The drawing under review shows one solid part. Ordinate dimensions are in mm from its lowest x, y, z. A direction names the side the tool comes from. Coordinates: 2 decimals unless noted, no trailing zeros. Order: outer loops, then holes, each group sorted by start corner. A loop starts at its lowest first (then second) coordinate and runs counter-clockwise, first axis right, second up. Notation, with made-up numbers: (88, -9.5) -> (101, -9.5) arc R27 ccw to (101, 7.5) -> close; hole circle Ø4 at (50.25, 45). An arc over 180 degrees is marked (long way). Write item = value, one per line.
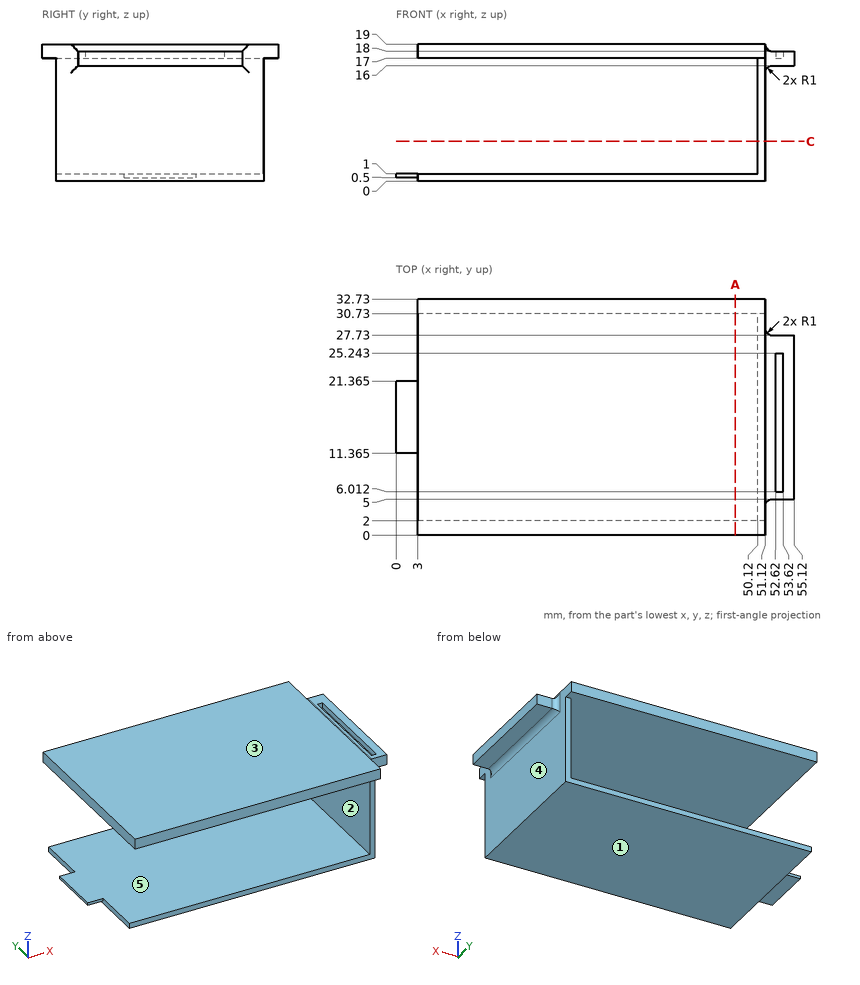
(1) For L1, parallel to Z at x = 11.5, y = 3; L2, parallel to X at y = 23.5, z = 7.75; L3, parallel to Z at x = 52, y = 14, list the stretches that pass through material, from the lowest coordinate up.
Report:
L1 = 0 to 1, 17 to 19
L2 = 50.12 to 51.12
L3 = 15.99 to 18.01
(2) For the marked faces 1 and 2, list the 3-axis set-ups (+Z, -Z, +X, -X, +Y, -Y) from which the entire face can be reached by the end or side of a thin tool; tool diameter is ignored.
Report:
face_1 = -Z, +X, -X, +Y, -Y
face_2 = -X, +Y, -Y
(3) Insertion check: pin 1 (1 mm diameter, centred on y = 21, z = 13.5, fed in from -X); pin 2 (0.5 mm diameter, centred on x = 53, z = 17.5, fed in from +Y); pin 3 (1.1 mm diameter, centred on x = 53, z = 17.5, fed in from -Y); pin 4 (4 mm diameter, centred on x = 17, y = 14.5, fed in from -Z). Each pin has a flat end and moves straight along its axis. Give the tip position at first contact, or say it passes through.
Report:
pin_1 = 50.12
pin_2 = 27.73
pin_3 = 5
pin_4 = 0
(4) The part is to be moulded in two halves that separate along Z. For the marked faces 3, 4 and 5, say which applies: released by +Z, released by -Z, zero draft, split by the parting line, or undercut.
Report:
face_3 = released by +Z
face_4 = zero draft
face_5 = undercut
(5) We need section C-C (z = 5.5). Write out the cut boundary in (x, y).
Report:
outline = (50.12, 2) -> (51.12, 2) -> (51.12, 30.73) -> (50.12, 30.73) -> close
(6) We need section A-A (x = 47). Write out the cut boundary in (y, z).
Report:
outline = (0, 17) -> (32.73, 17) -> (32.73, 19) -> (0, 19) -> close; (2, 0) -> (30.73, 0) -> (30.73, 1) -> (2, 1) -> close
